Input: part model. Units: mm. Frame: model coordinates. A direction names the side the tool comes from. Coordinates: 2 decimals unless noted, no trailing zeros. Loops run counter-clockwise (first coordinate to the right, second up) from the corner with the lowest first, then second, coordinate; pieces in that order, holes last. Notation, with made-up numbers: M 82.25,14 L 123.25,14 A19 cw 123.25,29 Z; hole C 74,-16.5 d3. An arc over 180 degrees is marked long. Use a Markdown table: item, result. Add a question column.
1. Pin query (flat end, axial travel): pin 1 (3 mm diameter, centred on y = 52.2, z = -158, fed in from -X); pin 2 (4 mm diameter, centred on x = 99, z = -158, fed in from -Y); pin 3 (6 mm diameter, centred on y = 30.5, z = -46.5, fed in from -X); pin 4 (4 mm diameter, centred on x = 3, z = -158, fed in from +Y). Return the tip coordinate at first contact, or that it passes through.
2. Set-up query: faces 1 (the flat face through (52, 10, 3)), 2 (the flat face through (105, 12, -82)). Return all of +Z, -Z, +X, -X, +Y, -Y with unobstructed straight access to the full face (end or side cutting, diameter ignored); none if empty.
3. Section B-B on x = 18. Output: boundary loops of the cut face in (y, z), then the cut area to 3 significant figures.
4. Line query: L1, parallel to X at y = -37.35, z = -158; L2, parallel to Y at x = 3, z = 0.5; L3, parallel to Z at x = 106, y = 52. Output: solid intervals per line, ascending. Write a range as [from, to].
5. Section A-A on z = -132.5. Output: boundary loops of the cut face in (x, y), then the cut area to 3 significant figures.
6. Draft query along Y for faces 3 (the cylindrical face through (105.79, 51.05, -4.75)), 4 (the flat face through (-3, -38, -81)), 5 (the cylindrical face through (2.49, 50.58, 0.79)), 6 (the flat face through (52, -40, -79)). Return one class per face: +Y half, -Y half, draft (parallel to the pull), parting line (faces both ways), or undercut.
```python
from build123d import *

# Parameters (mm, degrees)
SKETCH2_W                                      = 108
SKETCH2_H                                      = 95.2
BOSS_EXTRUDE1_DEPTH                            = 3
SKETCH3_W                                      = 167
SKETCH3_H                                      = 95.2
BOSS_EXTRUDE2_DEPTH                            = 3
SKETCH4_W                                      = 111
SKETCH4_H                                      = 167
BOSS_EXTRUDE3_DEPTH                            = 3
CSK_FOR_M3_FLAT_HEAD_MACHINE_SCREW1_AT_2_COUNT = 2
CSK_FOR_M3_FLAT_HEAD_MACHINE_SCREW1_AT_2_PITCH = 83.2
CSK_FOR_M3_FLAT_HEAD_MACHINE_SCREW2_AT_2_COUNT = 2
CSK_FOR_M3_FLAT_HEAD_MACHINE_SCREW2_AT_2_PITCH = 96
CSK_FOR_M3_FLAT_HEAD_MACHINE_SCREW3_AT_2_COUNT = 2
CSK_FOR_M3_FLAT_HEAD_MACHINE_SCREW3_AT_2_PITCH = 152
CUT_EXTRUDE1_REACH                             = 221.552
SKETCH12_W                                     = 6.5
SKETCH12_H                                     = 12
SKETCH12_W_2                                   = 6.2
SKETCH12_H_2                                   = 16
FILLET1_R                                      = 2
CHAMFER1_SIZE                                  = 2


with BuildPart() as part:
    # Sketch2 → Boss-Extrude1 (new body)
    with BuildSketch(Plane.XY):
        with Locations((51, 10.6)):
            Rectangle(SKETCH2_W, SKETCH2_H)
    extrude(amount=BOSS_EXTRUDE1_DEPTH)

    # Sketch3 → Boss-Extrude2 (add)
    with BuildSketch(Plane(origin=(105, 0, 0), x_dir=(0, 0, -1), z_dir=(1, 0, 0))):
        with Locations((80.5, 10.6)):
            Rectangle(SKETCH3_W, SKETCH3_H)
    extrude(amount=BOSS_EXTRUDE2_DEPTH)

    # Sketch4 → Boss-Extrude3 (add)
    with BuildSketch(Plane.XZ.offset(37)):
        with Locations((52.5, -80.5)):
            Rectangle(SKETCH4_W, SKETCH4_H)
    extrude(amount=BOSS_EXTRUDE3_DEPTH)

    # Sketch6 → CSK for M3 Flat Head Machine Screw1 (revolve, cut)
    with BuildSketch(Plane(origin=(3, -31, 3), x_dir=(0, -1, 0), z_dir=(1, 0, 0))):
        Polygon((0, 0), (0, 3), (1.7, 3), (1.7, 1.45), (3.15, 0), align=None)
    csk_for_m3_flat_head_machine_screw1 = revolve(axis=Axis((3, -31, 9.35), (0, 0, -1)), mode=Mode.SUBTRACT)

    # CSK for M3 Flat Head Machine Screw1 at 2: CSK for M3 Flat Head Machine Screw1 ×2
    with Locations(*[(0, i * CSK_FOR_M3_FLAT_HEAD_MACHINE_SCREW1_AT_2_PITCH, 0) for i in range(1, CSK_FOR_M3_FLAT_HEAD_MACHINE_SCREW1_AT_2_COUNT)]):
        add(csk_for_m3_flat_head_machine_screw1, mode=Mode.SUBTRACT)

    # Sketch8 → CSK for M3 Flat Head Machine Screw2 (revolve, cut)
    with BuildSketch(Plane(origin=(3, -40, -158), x_dir=(0, 0, -1), z_dir=(1, 0, 0))):
        Polygon((0, 0), (0, 3), (1.7, 3), (1.7, 1.45), (3.15, 0), align=None)
    csk_for_m3_flat_head_machine_screw2 = revolve(axis=Axis((3, -46.35, -158), (0, 1, 0)), mode=Mode.SUBTRACT)

    # CSK for M3 Flat Head Machine Screw2 at 2: CSK for M3 Flat Head Machine Screw2 ×2
    with Locations(*[(i * CSK_FOR_M3_FLAT_HEAD_MACHINE_SCREW2_AT_2_PITCH, 0, 0) for i in range(1, CSK_FOR_M3_FLAT_HEAD_MACHINE_SCREW2_AT_2_COUNT)]):
        add(csk_for_m3_flat_head_machine_screw2, mode=Mode.SUBTRACT)

    # Sketch10 → CSK for M3 Flat Head Machine Screw3 (revolve, cut)
    with BuildSketch(Plane(origin=(108, 52.2, -6), x_dir=(0, 0, -1), z_dir=(0, 1, 0))):
        Polygon((0, 0), (0, 3), (1.7, 3), (1.7, 1.45), (3.15, 0), align=None)
    csk_for_m3_flat_head_machine_screw3 = revolve(axis=Axis((114.35, 52.2, -6), (-1, 0, 0)), mode=Mode.SUBTRACT)

    # CSK for M3 Flat Head Machine Screw3 at 2: CSK for M3 Flat Head Machine Screw3 ×2
    with Locations(*[(0, 0, -i * CSK_FOR_M3_FLAT_HEAD_MACHINE_SCREW3_AT_2_PITCH) for i in range(1, CSK_FOR_M3_FLAT_HEAD_MACHINE_SCREW3_AT_2_COUNT)]):
        add(csk_for_m3_flat_head_machine_screw3, mode=Mode.SUBTRACT)

    # Sketch12 → Cut-Extrude1 (cut, up to next)
    with BuildSketch(Plane.XZ.offset(40), mode=Mode.PRIVATE) as cut_extrude1_sk1:
        with Locations((41.25, -15.5)):
            Rectangle(SKETCH12_W, SKETCH12_H)
    cut_extrude1_tool1 = extrude(cut_extrude1_sk1.sketch, amount=-CUT_EXTRUDE1_REACH, mode=Mode.PRIVATE) & part.part
    # Sketch12 → Cut-Extrude1 (cut, up to next)
    with BuildSketch(Plane.XZ.offset(40), mode=Mode.PRIVATE) as cut_extrude1_sk2:
        with Locations((86.5, -17.5)):
            Rectangle(SKETCH12_W_2, SKETCH12_H_2)
    cut_extrude1_tool2 = extrude(cut_extrude1_sk2.sketch, amount=-CUT_EXTRUDE1_REACH, mode=Mode.PRIVATE) & part.part
    # Sketch12 → Cut-Extrude1 (cut, up to next)
    with BuildSketch(Plane.XZ.offset(40), mode=Mode.PRIVATE) as cut_extrude1_sk3:
        with Locations((86.5, -143.5)):
            Rectangle(SKETCH12_W_2, SKETCH12_H_2)
    cut_extrude1_tool3 = extrude(cut_extrude1_sk3.sketch, amount=-CUT_EXTRUDE1_REACH, mode=Mode.PRIVATE) & part.part
    # Sketch12 → Cut-Extrude1 (cut, up to next)
    with BuildSketch(Plane.XZ.offset(40), mode=Mode.PRIVATE) as cut_extrude1_sk4:
        with Locations((41.25, -145.5)):
            Rectangle(SKETCH12_W, SKETCH12_H)
    cut_extrude1_tool4 = extrude(cut_extrude1_sk4.sketch, amount=-CUT_EXTRUDE1_REACH, mode=Mode.PRIVATE) & part.part
    add(cut_extrude1_tool1.solids().sort_by_distance((41.25, -40, -15.5))[0], mode=Mode.SUBTRACT)
    add(cut_extrude1_tool2.solids().sort_by_distance((86.5, -40, -17.5))[0], mode=Mode.SUBTRACT)
    add(cut_extrude1_tool3.solids().sort_by_distance((86.5, -40, -143.5))[0], mode=Mode.SUBTRACT)
    add(cut_extrude1_tool4.solids().sort_by_distance((41.25, -40, -145.5))[0], mode=Mode.SUBTRACT)

    # Fillet1
    fillet1_edges = [part.edges().sort_by_distance(p)[0] for p in [
        (44.5, -38.5, -139.5),
        (44.5, -38.5, -151.5),
        (38, -38.5, -151.5),
        (38, -38.5, -139.5),
        (89.6, -38.5, -135.5),
        (89.6, -38.5, -151.5),
        (83.4, -38.5, -151.5),
        (83.4, -38.5, -135.5),
        (83.4, -38.5, -9.5),
        (89.6, -38.5, -9.5),
        (89.6, -38.5, -25.5),
        (83.4, -38.5, -25.5),
        (38, -38.5, -9.5),
        (44.5, -38.5, -9.5),
        (44.5, -38.5, -21.5),
        (38, -38.5, -21.5),
    ]]
    fillet(fillet1_edges, radius=FILLET1_R)

    # Chamfer1
    chamfer1_edges = [part.edges().sort_by_distance(p)[0] for p in [
        (105, -37, -82),
        (105, 10.6, 0),
        (51, -37, 0),
    ]]
    chamfer(chamfer1_edges, length=CHAMFER1_SIZE)


solid = part.part
```
Answers below:
| question | item | result |
|---|---|---|
| 1 | pin 1 | passes through |
| 1 | pin 2 | stops at y = -38.85 |
| 1 | pin 3 | stops at x = 105 |
| 1 | pin 4 | stops at y = -37 |
| 2 | face 1 | +Z, +X, -X, +Y, -Y |
| 2 | face 2 | -Z, -X, +Y |
| 3 | outline | M -40,-164 L -37,-164 L -37,-2 L -35,0 L 58.2,0 L 58.2,3 L -40,3 Z |
| 3 | area | 789 mm² |
| 4 | L1 | x = [-3, 1.3], [4.7, 97.3], [100.7, 108] |
| 4 | L2 | y = [-40, -32.7], [-29.3, 50.5], [53.9, 58.2] |
| 4 | L3 | z = [-164, -159.69], [-156.31, -7.69], [-4.31, 3] |
| 5 | outline | M -3,-40 L 108,-40 L 108,58.2 L 105,58.2 L 105,-35 L 103,-37 L -3,-37 Z |
| 5 | area | 621 mm² |
| 6 | face 3 | undercut |
| 6 | face 4 | draft |
| 6 | face 5 | undercut |
| 6 | face 6 | -Y half |
